```python
from build123d import *

# Parameters (mm, degrees)
ESBO_O1_R                = 15
RESSALTO_EXTRUS_O1_DEPTH = 10


with BuildPart() as part:
    # Esboço1 → Ressalto-extrusão1 (new body)
    with BuildSketch(Plane(origin=(0, 0, 0), x_dir=(1, 0, 0), z_dir=(0, 1, 0))):
        with Locations(Location((0, 0, 0), (0, 0, 270))):
            Circle(ESBO_O1_R)
        with BuildLine():
            Line((1.05, -1), (1.05, 1))
            ThreePointArc((1.05, 1), (-1.45, 0), (1.05, -1))
        make_face(mode=Mode.SUBTRACT)
        with BuildLine():
            Line((1.20846299, -5.78116293), (1.861701017, -11.094889334))
            ThreePointArc((1.861701017, -11.094889334), (8.142596912, -7.762771124), (11.171107828, -1.329981166))
            Line((11.171107828, -1.329981166), (5.865248184, -0.693607497))
            ThreePointArc((5.865248184, -0.693607497), (4.356621686, -3.987740601), (1.20846299, -5.78116293))
        make_face(mode=Mode.SUBTRACT)
        with BuildLine():
            Line((-5.78116293, -1.20846299), (-11.094889334, -1.861701017))
            ThreePointArc((-11.094889334, -1.861701017), (-7.762771124, -8.142596912), (-1.329981166, -11.171107828))
            Line((-1.329981166, -11.171107828), (-0.693607497, -5.865248184))
            ThreePointArc((-0.693607497, -5.865248184), (-3.987740601, -4.356621686), (-5.78116293, -1.20846299))
        make_face(mode=Mode.SUBTRACT)
        with BuildLine():
            Line((-1.20846299, 5.78116293), (-1.861701017, 11.094889334))
            ThreePointArc((-1.861701017, 11.094889334), (-8.142596912, 7.762771124), (-11.171107828, 1.329981166))
            Line((-11.171107828, 1.329981166), (-5.865248184, 0.693607497))
            ThreePointArc((-5.865248184, 0.693607497), (-4.356621686, 3.987740601), (-1.20846299, 5.78116293))
        make_face(mode=Mode.SUBTRACT)
        with BuildLine():
            Line((5.78116293, 1.20846299), (11.094889334, 1.861701017))
            ThreePointArc((11.094889334, 1.861701017), (7.762771124, 8.142596912), (1.329981166, 11.171107828))
            Line((1.329981166, 11.171107828), (0.693607497, 5.865248184))
            ThreePointArc((0.693607497, 5.865248184), (3.987740601, 4.356621686), (5.78116293, 1.20846299))
        make_face(mode=Mode.SUBTRACT)
    extrude(amount=RESSALTO_EXTRUS_O1_DEPTH)


solid = part.part
```
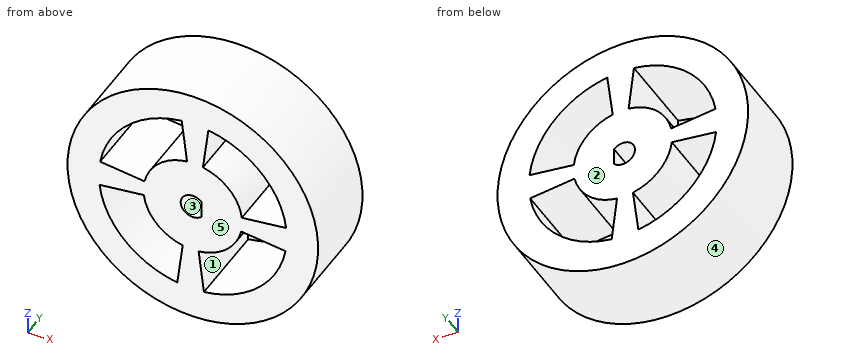
Check sheet for the modelled part. Datum: model origin and axes. Units: mm. Face numbers are marked on the shaded views. A direction names the side the tool comes from. Round coordinates to 2 decimals unless told otherwise and drop trailing zeros. Write each loop counter-clockwise with the first axis right and the second up, starting at its lowest first coordinate (ties: lowest second). Pieces come first, ordered by that corner, then holes. Notation, with made-up numbers: (81, 15.25) -> (130, 15.25) arc R32 ccw to (130, 44.25) -> close; hole circle Ø2 at (69.25, -23.75). An arc over 180 degrees is marked (long way). One line per question, with ' | ' between items. Start each with the question number.
1. Scan lines: line 1 along Z through (x, y) = (-9.25, 4.25); line 2 along X through (y, z) = (8.25, 0); line 3 along X through (y, z) = (5, -3.25). Record each from-to range of solid material in increasing order. Write a range as from..to.
2. Sectioned sample at B-B, the plane z = 0. Record the cut outline in (x, y).
3. Depth check by flat-ended pin: pin 1 (5 mm diameter, centred on x = 8, y = 7.5, fed in from +Z); pin 2 (6 mm diameter, centred on y = 3, z = 5, fed in from +X). Enter the tip coordinate at first touch or a pass-through.
4. Sectioned sample at C-C, the plane y = 3. Record the cut outline in (x, z).
5. Set-up check for the marked faces 1 and 2: record each of +Z, -Z, +X, -X, +Y, -Y from which the full face is reachable in a straight line by a thin tool's end or side.
6. Sectioned sample at A-A, the plane x = 0. Record the cut outline in (y, z).
7. Release check for a two-part mould opening along Z. For the marked faces 3, 4 and 5 record: +Z half, -Z half, draft (parallel to the pull), parting line (faces both ways), or undercut.
8. Sectioned sample at D-D, the plane z = -5.25. Record the cut outline in (x, y), then the cut area to 3 significant figures.
Taken from the geometry:
1) line 1: z = -11.81..-6.4, -1.1..1.63, 6.4..11.81 | line 2: x = -15..-1.45, 1.05..15 | line 3: x = -14.64..-10.77, -4.93..4.93, 10.77..14.64
2) outline: (-15, 0) -> (-1.45, 0) -> (-1.45, 10) -> (-15, 10) -> close; (1.05, 0) -> (15, 0) -> (15, 10) -> (1.05, 10) -> close
3) pin 1: stops at z = 13.96 | pin 2: stops at x = 14.87
4) outline: circle Ø30 at (0, 0); hole (-11.17, -1.33) arc R11.25 ccw to (-1.86, -11.09) -> (-1.21, -5.78) arc R5.91 cw to (-5.87, -0.69) -> close; hole (-11.09, 1.86) -> (-5.78, 1.21) arc R5.91 cw to (-0.69, 5.87) -> (-1.33, 11.17) arc R11.25 ccw to start; hole (0.69, -5.87) -> (1.33, -11.17) arc R11.25 ccw to (11.09, -1.86) -> (5.78, -1.21) arc R5.91 cw to start; hole (1.05, -1) -> (1.05, 1) arc R1.45 ccw (long way) to start; hole (1.21, 5.78) arc R5.91 cw to (5.87, 0.69) -> (11.17, 1.33) arc R11.25 ccw to (1.86, 11.09) -> close
5) face 1: +Y, -Y | face 2: +Z, -Z, +X, -X, +Y
6) outline: (0, -15) -> (10, -15) -> (10, -1.45) -> (0, -1.45) -> close; (0, 1.45) -> (10, 1.45) -> (10, 15) -> (0, 15) -> close
7) face 3: undercut | face 4: parting line | face 5: draft
8) outline: (-14.05, 0) -> (-9.95, 0) -> (-9.95, 10) -> (-14.05, 10) -> close; (-2.71, 0) -> (2.71, 0) -> (2.71, 10) -> (-2.71, 10) -> close; (9.95, 0) -> (14.05, 0) -> (14.05, 10) -> (9.95, 10) -> close | area: 136 mm^2
